from build123d import *

# Parameters (mm, degrees)
F0_R     = 19.05
F1_DEPTH = 12.7
F2_R     = 12.573
F3_DEPTH = 50.8


with BuildPart() as f1:
    # F0 (on Right) → F1 (new body)
    with BuildSketch(Plane.YZ):
        Circle(F0_R)
    extrude(amount=F1_DEPTH)

    # F2 (on face) → F3 (join)
    with BuildSketch(Plane.YZ.offset(12.7)):
        Circle(F2_R)
    extrude(amount=F3_DEPTH)

    # F5 (on offset) → F6 (revolve, cut)
    with BuildSketch(Plane.YZ.offset(69.85)):
        with BuildLine():
            Line((-12.573, 0), (12.573, 0))
            ThreePointArc((12.573, 0), (0, 12.573), (-12.573, 0))
        make_face()
    revolve(axis=Axis((69.85, 16.413388, 0), (0, 1, 0)), mode=Mode.SUBTRACT)


solid = f1.part
Read the model definition and answer for the solid it produces. Units are mm, in the model's axes. A direction names the side the tool comes from. Coordinates: 2 decimals unless noted, no trailing zeros. Write each loop counter-clockwise with the first axis right and the second up, starting at its lowest first coordinate (ties: lowest second). Pieces come first, ordered by that corner, then holes. Notation, with made-up numbers: (-31, -15) -> (-20, -15) arc R12 ccw to (-20, -4) -> close; hole circle Ø1 at (21, 46). An arc over 180 degrees is marked (long way). Return JSON: item names as keys, results as strings.
(1) The part is cut by section D-D on x = 11. Give the vertices of the cut face in (y, z).
Answers below:
{"outline": "circle Ø38.1 at (0, 0)"}
(2) Which of the six approach directions +Z, -Z, +X, -X, +Y, -Y give full straight-line access (tool end or side, diameter ignored) to faces 1 (the flat face through (12.7, 4, -12.4)), 2 (the flat face through (63.5, -11.2, 0.1))?
Answers below:
{"face 1": "+X", "face 2": "+Z, -Z, +X, +Y, -Y"}
(3) The part is cut by section A-A on z = 0. Give the vertices of the cut face in (x, y).
Answers below:
{"outline": "(0, -19.05) -> (12.7, -19.05) -> (12.7, -12.57) -> (63.5, -12.57) -> (63.5, -10.85) arc R12.57 cw to (63.5, 10.85) -> (63.5, 12.57) -> (12.7, 12.57) -> (12.7, 19.05) -> (0, 19.05) -> close"}
(4) The part is cut by section C-C on x = 50. Give the vertices of the cut face in (y, z), then the cut area to 3 significant figures.
Answers below:
{"outline": "circle Ø25.15 at (0, 0)", "area": "497 mm^2"}
(5) Consider line 1 along X through (y, z) = (12.5, 9.5); line 2 along Y through (x, z) = (27, 9); line 3 along Z through (x, y) = (7.5, -10). Determine where each line is inside the solid, lowest interval first. Write a range as from..to.
Answers below:
{"line 1": "0..12.7", "line 2": "-8.78..8.78", "line 3": "-16.21..16.21"}
(6) Each of these flat-tipped pins is pushed along its axis until it touches: P1, Ø3, axis at y = 5.5, z = -4, coming from the +X side; P2, Ø5, axis at x = 41.5, z = -7, coming from the -Y side; P3, Ø10, axis at x = 10, y = -1.5, coming from the +Z side. Where does it stop, or does it pass through?
Answers below:
{"P1": "x = 60.41", "P2": "y = -11.74", "P3": "z = 19.05"}
